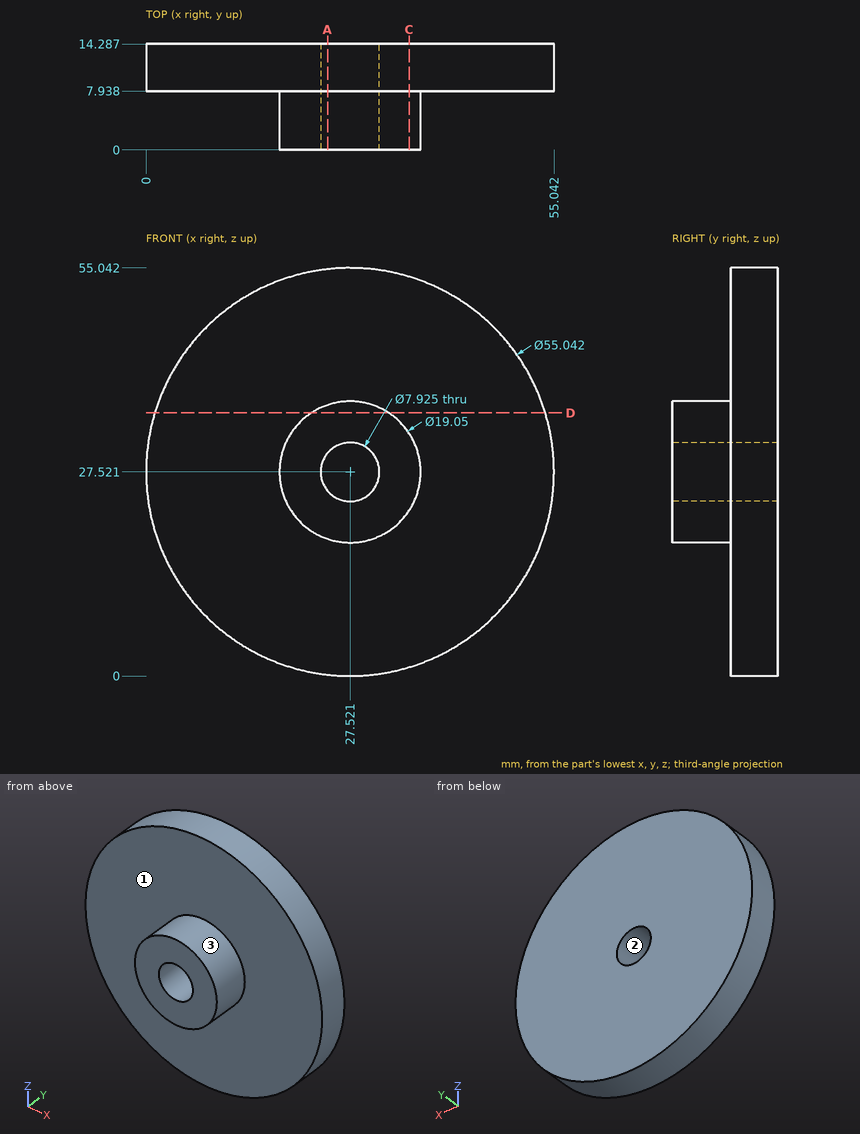
Drawing for the job (mm, zero at the part's lowest x, y, z). Give positions to 0.01 mm unless a question says otherwise; leave off trailing zeros. Loops run counter-clockwise (first coordinate to the right, second up) from the corner with the lowest first, then second, coordinate; pieces in that order, holes last.
(1) Drill centre lines: line 1 along Y through (x, z) = (14, 36); line 2 along X through (y, z) = (1.75, 24) (1 decimal); line 3 along Z through (x, y) = (27, 3.25). Where is each one in solid material? Low to high.
Return value:
line 1: y = 7.94 to 14.29
line 2: x = 18.7 to 25.7, 29.3 to 36.4
line 3: z = 18.01 to 23.59, 31.45 to 37.03
(2) Band-saw the part on A-A (x = 24.5). Write the cut outline in (y, z) (1 decimal).
Return value:
outline: (0, 18.5) - (7.9, 18.5) - (7.9, 0.2) - (14.3, 0.2) - (14.3, 25) - (0, 25) - close; (0, 30.1) - (14.3, 30.1) - (14.3, 54.9) - (7.9, 54.9) - (7.9, 36.6) - (0, 36.6) - close
(3) Pull direction Z, two halves, no side cores. Call the marked faces 1, 2 and 3: pulls with the +Z half, pulls with the -Z half, needs draft (parallel to the pull), parting line crosses it, or undercut.
Return value:
face 1: needs draft
face 2: undercut
face 3: parting line crosses it
(4) Band-saw the part on C-C (x = 35.5). Write the cut outline in (y, z).
Return value:
outline: (0, 22.32) - (7.94, 22.32) - (7.94, 1.18) - (14.29, 1.18) - (14.29, 53.86) - (7.94, 53.86) - (7.94, 32.72) - (0, 32.72) - close
(5) Pin check, flat tips, straight feed: pin 1 (4 mm diameter, centred on y = 8, z = 26.5, fed in from -X); pin 2 (1 mm diameter, centred on x = 15.5, y = 9, fed in from -Z); pin 3 (5 mm diameter, centred on y = 2.5, z = 32.5, fed in from -X) (1 decimal); pin 4 (6 mm diameter, centred on x = 23, y = 11, fed in from -Z). Stop position of each tip, or through.
Return value:
pin 1: stops at x = 0
pin 2: stops at z = 2.53
pin 3: stops at x = 18.3
pin 4: stops at z = 0.04
(6) Band-saw the part on D-D (z = 35.5). Write the cut outline in (x, y).
Return value:
outline: (1.18, 7.94) - (22.32, 7.94) - (22.32, 0) - (32.72, 0) - (32.72, 7.94) - (53.86, 7.94) - (53.86, 14.29) - (1.18, 14.29) - close
